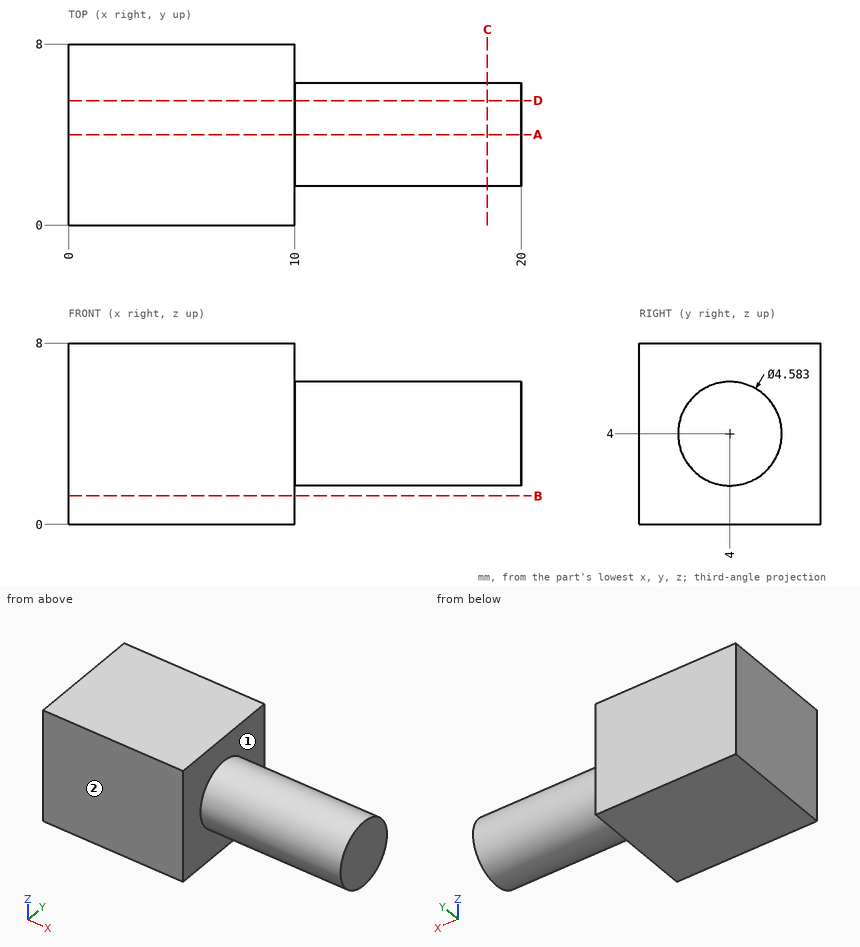
Job drawing, mm, ordinate dimensions from the low corner. One solid piece. A direction names the side the tool comes from. Give positions to 0.01 mm unless a question says otherwise; leave off trailing zeros. Loops run counter-clockwise (first coordinate to the right, second up) from the corner with the lowest first, then second, coordinate; pieces in that order, holes last. Notation, with made-up numbers: M -7,67.5 L 33,67.5 A25 cw 33,101.5 Z; hole C -14,-25.75 d3. An arc over 180 degrees is marked long. Return JSON: item names as keys, results as strings.
1) 3-axis set-ups, long thin cutter, end or side, ignore diameter. For the marked faces 1 and 2: which of +Z, -Z, +X, -X, +Y, -Y reach the whole face in a straight line?
Calculated:
{"face 1": "+X", "face 2": "+Z, -Z, +X, -X, -Y"}
2) Saw through at D-D, the plane y = 5.5. List the corners of the cut face in (x, z).
Calculated:
{"outline": "M 0,0 L 10,0 L 10,2.27 L 20,2.27 L 20,5.73 L 10,5.73 L 10,8 L 0,8 Z"}
3) Drill centre lines: line 1 (X direction, y = 4.75, z = 6.25); line 2 (Z direction, x = 10.5, y = 4.5); line 3 (Z direction, x = 12.75, y = 2) (1 decimal). Where is each one in solid material? Low to high.
Calculated:
{"line 1": "x = 0 to 10", "line 2": "z = 1.76 to 6.24", "line 3": "z = 2.9 to 5.1"}
4) Saw through at C-C, the plane x = 18.5. List the corners of the cut face in (y, z).
Calculated:
{"outline": "C 4,4 d4.58"}
5) Saw through at B-B, the plane z = 1.25. List the corners of the cut face in (x, y).
Calculated:
{"outline": "M 0,0 L 10,0 L 10,8 L 0,8 Z"}
6) Saw through at A-A, the plane y = 4. List the corners of the cut face in (x, z).
Calculated:
{"outline": "M 0,0 L 10,0 L 10,1.71 L 20,1.71 L 20,6.29 L 10,6.29 L 10,8 L 0,8 Z"}
7) Flat gauge pins, fed straight in: pin 1 Ø4 at (x, z) = (3, 2) entering from -Y; pin 2 Ø1 at (y, z) = (5, 1) entering from +X; pin 3 Ø1.5 at (x, y) = (16, 4.5) entering from -Z. Where does each tip first touch, or does it go through?
Calculated:
{"pin 1": "stops at y = 0", "pin 2": "stops at x = 10", "pin 3": "stops at z = 1.71"}
